Geometry: final body of the model. Coordinates: model frame, mm. Face numbers are marked on the shaded views. A direction names the side the tool comes from. Give positions to 0.01 mm unless a question says otherwise; leave off trailing zeros. Order: outer loops, then holes, each group sorted by start corner. A loop starts at its lowest first (then second) coordinate and runs counter-clockwise, first axis right, second up. Notation, with made-up numbers: (80.25, 2.5) - (111.25, 2.5) arc R33 cw to (111.25, 37.5) - close; hole circle Ø8 at (-0.5, 76.25). An arc over 180 degrees is marked (long way). One line per item, written item: value.
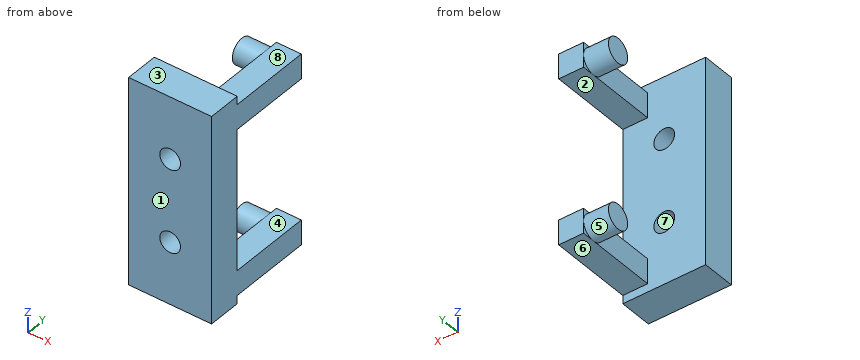
Autodesk Inventor part; units mm, degrees
ref_plane "YZ Plane" through (0, 0, 0) normal (1, 0, 0) x (0, 1, 0)
ref_plane "XZ Plane" through (0, 0, 0) normal (0, 1, 0) x (-1, 0, 0)
ref_plane "XY Plane" through (0, 0, 0) normal (0, 0, 1) x (1, 0, 0)
sketch "Sketch1" plane through (0, 0, 0) normal (0, 1, 0) x (-1, 0, 0)
  line L0 (0, 0) -> (10, 0)
  line L1 (10, 0) -> (10, -25)
  line L2 (10, -25) -> (0, -25)
  line L3 (0, -25) -> (0, 0)
  dimension "d0" = 10
  dimension "d1" = 25
extrude "Extrusion1" add sketch "Sketch1" along normal blind 4
sketch "Sketch2" plane through (0, 4, 0) normal (0, 1, 0) x (1, 0, 0)
  line L0 (0, 0) -> (0, 12.5)
  line L1 (0, 0) -> (0, 25)
  line L2 (0, 12.5) -> (0, 7.5)
  line L3 (0, 12.5) -> (0, 17.5)
  line L4 (0, 17.5) -> (-5, 17.5)
  line L5 (-10, 25) -> (-10, 0)
  circle A0 centre (-5, 17.5) radius 1.25
  line L6 (0, 7.5) -> (-5, 7.5)
  circle A1 centre (-5, 7.5) radius 1.25
  dimension "d4" = 12.5
  dimension "d5" = 5
  dimension "d6" = 5
  dimension "d7" = 5
  dimension "d8" = 2.5
  dimension "d9" = 5
  dimension "d10" = 2.5
extrude "Extrusion2" cut sketch "Sketch2" against normal blind 5
sketch "Sketch3" plane through (0, 4, 0) normal (0, 1, 0) x (1, 0, 0)
  line L0 (0, 25) -> (0, 0)
  line L1 (0, 25) -> (0, 24)
  line L2 (0, 24) -> (-3, 24)
  line L3 (-3, 24) -> (-3, 21)
  line L4 (-3, 21) -> (0, 21)
  line L5 (0, 21) -> (0, 24)
  line L6 (0, 0) -> (0, 1)
  line L7 (0, 1) -> (-3, 1)
  line L8 (-3, 1) -> (-3, 4)
  line L9 (-3, 4) -> (0, 4)
  line L10 (0, 4) -> (0, 1)
  dimension "d13" = 1
  dimension "d14" = 3
  dimension "d15" = 3
  dimension "d16" = 1
  dimension "d17" = 3
  dimension "d18" = 3
extrude "Extrusion3" add sketch "Sketch3" along normal blind 10
sketch "Sketch4" plane through (-3, 4, -24) normal (-1, 0, 0) x (0, 0, 1)
  line L0 (0, 0) -> (0, 10)
  line L1 (0, 10) -> (1.5, 10)
  line L2 (1.5, 10) -> (1.5, 8.5)
  line L3 (1.5, 8.5) -> (0, 8.5)
  line L4 (0, 8.5) -> (0, 10)
  circle A0 centre (1.5, 8.5) radius 1.5
  line L5 (23, 10) -> (20, 10)
  line L6 (23, 10) -> (21.5, 10)
  line L7 (21.5, 10) -> (21.5, 8.5)
  line L8 (21.5, 8.5) -> (23, 8.5)
  line L9 (23, 8.5) -> (23, 10)
  circle A1 centre (21.5, 8.5) radius 1.5
  point P0 (24, -4)
  dimension "d21" = 1.5
  dimension "d22" = 1.5
  dimension "d23" = 3
  dimension "d24" = 1.5
  dimension "d25" = 1.5
  dimension "d26" = 3
extrude "Extrusion4" add sketch "Sketch4" along normal blind 3 contours A0 L2 L3 | L3 L2 A0 | A1 L8 L7 | L7 L8 A1
properties part number "LaserMount"
1) First-contact query: pin 1 (0.9 mm diameter, centred on x = -1, y = 11.5, fed in from -Z); pin 2 (2 mm diameter, centred on x = -2, z = -18.5, fed in from +Y); pin 3 (2.5 mm diameter, centred on y = 10.5, z = -2.5, fed in from -X); pin 4 (2 mm diameter, centred on x = -5.5, y = 6, fed in from -Z). Flat tips, straight axial feed; report the tip coordinate or a pass-through.
Answers below:
pin 1: z = -24
pin 2: y = 4
pin 3: x = -6
pin 4: through
2) Section D-D, the plane y = 1.25. Return loops of the section in (x, z).
Answers below:
outline: (-10, -25) - (0, -25) - (0, 0) - (-10, 0) - close; hole circle Ø2.5 at (-5, -17.5); hole circle Ø2.5 at (-5, -7.5)
3) Section C-C, the plane x = -3.5. Return loops of the section in (y, z).
Answers below:
outline: (0, -25) - (4, -25) - (4, 0) - (0, 0) - close; circle Ø3 at (12.5, -22.5); circle Ø3 at (12.5, -2.5)
4) Material intervals for line 1 along Z through (x, y) = (-5, 0.9); line 2 along X through (y, z) = (1.05, -17.5); line 3 along Z through (x, y) = (-0.75, 10.5), sorted ascending.
Answers below:
line 1: -25 to -18.75, -16.25 to -8.75, -6.25 to 0
line 2: -10 to -6.25, -3.75 to 0
line 3: -24 to -21, -4 to -1
5) Mould query, pull axis Z, two halves, no side actions, for the marked faces 1, 2 and 3. Classes: released by +Z, released by -Z, zero draft, split by the parting line, or undercut.
Answers below:
face 1: zero draft
face 2: undercut
face 3: released by +Z
6) Section A-A, the plane z = -18.5. Return loops of the section in (x, y), then the cut area to 3 significant figures.
Answers below:
outline: (-10, 0) - (-5.75, 0) - (-5.75, 4) - (-10, 4) - close; (-4.25, 0) - (0, 0) - (0, 4) - (-4.25, 4) - close
area: 34.0 mm^2
7) Section B-B, the plane y = 4.25. Return loops of the section in (x, z), then the cut area to 3 significant figures.
Answers below:
outline: (-3, -24) - (0, -24) - (0, -21) - (-3, -21) - close; (-3, -4) - (0, -4) - (0, -1) - (-3, -1) - close
area: 18.0 mm^2
8) Set-up query: the marked faces 4, 5, 6, 7 and 8. Return all of +Z, -Z, +X, -X, +Y, -Y with unobstructed straight access to the full face (end or side cutting, diameter ignored); none if empty.
Answers below:
face 4: +X, -X, +Y
face 5: -X
face 6: -Z, +X, -X, +Y
face 7: +Y, -Y
face 8: +Z, +X, -X, +Y
